The model under review builds one solid part; all positions refer to its coordinate system, in mm. A direction names the side the tool comes from. Coordinates: 2 decimals unless noted, no trailing zeros. Order: outer loops, then holes, each group sorted by start corner. A loop starts at its lowest first (then second) coordinate and runs counter-clockwise, first axis right, second up. Notation, with made-up numbers: M 2,71 L 49,71 A24 cw 49,97 Z; hole C -36.5,18.25 d6. An arc over 180 degrees is marked long. One line per item, written item: value.
Autodesk Inventor part; units mm, degrees
ref_plane "Offsets" through (0, 0, 50) normal (0, 0, 1) x (1, 0, 0)
ref_plane "Work Plane3" through (0, 17, 100) normal (0, 1, 0) x (-1, 0, 0)
ref_plane "YZ Plane" through (0, 0, 0) normal (1, 0, 0) x (0, 1, 0)
ref_plane "Offsets" through (0, 0, 50) normal (0, 0, 1) x (1, 0, 0)
ref_plane "Work Plane4" through (0, 0, 25) normal (0, 0, 1) x (1, 0, 0)
sketch "Sketch1" plane through (0, 0, 0) normal (0, 0, 1) x (1, 0, 0)
  circle A0 centre (0, 0) radius 19.0246
  dimension "d0" = 38.0492
extrude "Extrusion1" add sketch "Sketch1" along normal blind 100
sketch "Sketch2" plane through (0, 0, 100) normal (0, 0, 1) x (1, 0, 0)
  circle A0 centre (0, 0) radius 19.0246
  circle A1 centre (0, 0) radius 17
  dimension "d3" = 34
extrude "Extrusion2" cut sketch "Sketch2" against normal up to surface (75 mm away)
sketch "Sketch8" plane through (0, 0, 100) normal (0, 0, 1) x (1, 0, 0)
  circle A0 centre (0, 0) radius 17
  circle A1 centre (0, 0) radius 12.5
  dimension "d75" = 25
extrude "Extrusion7" cut sketch "Sketch8" against normal up to surface (50 mm away)
sketch "Sketch3" plane through (0, 0, 0) normal (0, 0, -1) x (-1, 0, 0)
  circle A0 centre (0, 0) radius 19.0246
hole "Hole1" at (0, 0, 0) direction (0, 0, 1) diameter 12 depth 50 tip angle 118
sketch "Sketch4" plane through (0, 0, 0) normal (0, 1, 0) x (-1, 0, 0)
  line L0 (-19.0246, 0) -> (19.0246, 0)
  line L1 (3.25, 44.15) -> (3.25, 30.65)
  line L2 (-3.25, 30.65) -> (-3.25, 44.15)
  arc A0 (-3.25, 30.65) -> (3.25, 30.65) centre (0, 30.65) ccw
  arc A1 (3.25, 44.15) -> (-3.25, 44.15) centre (0, 44.15) ccw
  line L3 (0, -9.83) -> (0, 58.98)
  line L4 (-5, 44.15) -> (-5, 30.65)
  arc A2 (-5, 30.65) -> (5, 30.65) centre (0, 30.65) ccw
  line L5 (5, 30.65) -> (5, 44.15)
  arc A3 (5, 44.15) -> (-5, 44.15) centre (0, 44.15) ccw
  point P0 (-19.0246, 25.4)
  point P1 (19.0246, 25.4)
  dimension "d13" = 6.5
  dimension "d15" = 20
  dimension "d76" = 5
extrude "Extrusion3" cut sketch "Sketch4" along normal through all both and the other way through all contours L1 A0 L3 A1 | L3 A0 L2 A1
sketch "Sketch9" plane through (0, 0, 0) normal (0, 0, -1) x (-1, 0, 0)
  circle A0 centre (0, 0) radius 19.0246
  circle A1 centre (0, 0) radius 12.7 construction
  point P0 (-12.7, 0)
  dimension "d49" = 25.4
hole "Hole3" at (12.7, 0, 0) direction (0, 0, 1) diameter 3.937 depth 19.05 tip angle 118
pattern_circular "Circular Pattern1" count 4 over 360 about axis through (0, 0, 25) along (0, 0, -1) of "Hole3"
ref_plane "Work Plane3" through (0, 17, 100) normal (0, 1, 0) x (-1, 0, 0)
extrude "Extrusion12" cut sketch "Sketch4" against normal blind 5 from surface at 17
sketch "Sketch12" plane through (0, 0, 100) normal (0, 0, 1) x (1, 0, 0)
  circle A0 centre (0, 0) radius 10
  circle A1 centre (0, 0) radius 9
  line L0 (-3.0902, 9.5106) -> (-3.0902, 8.4529) construction
  line L1 (3.0902, 9.5106) -> (3.0902, 8.4529) construction
  line L2 (-3.0902, 9.5106) -> (0, 0)
  line L3 (0, 0) -> (3.0902, 9.5106)
  point P0 (2.7812, 8.5595)
  point P1 (-2.7812, 8.5595)
  dimension "d85" = 20
  dimension "d98" = 18
  dimension "d112" = 36
sketch "Sketch15" plane through (0, 0, 100) normal (0, 0, 1) x (1, 0, 0)
  circle A0 centre (0, 0) radius 12
  circle A1 centre (0, 0) radius 12.5
  dimension "d113" = 24
extrude "Extrusion15" cut sketch "Sketch15" against normal blind 12
thread "Thread1"
extrude "Extrusion13" add sketch "Sketch12" along normal blind 14.5 contours L3 L2 A1 | A1 L2 L3
extrude "Extrusion14" add sketch "Sketch12" along normal up to surface (14.5 mm away) contours L3 A1 L2 A0 picked at (1.6921, 9.4688)
pattern_circular "Circular Pattern2" count 5 over 360 about axis through (0, 0, -10) along (0, 0, 1) of "Extrusion14"
sketch "Sketch14" plane through (0, 0, 114.5) normal (0, 0, 1) x (1, 0, 0)
  point P0 (0, 0)
  point P1 (0, 0)
  point P2 (0, 0)
hole "Hole6" at (0, 0, 114.5) direction (0, 0, -1) diameter 6.647 depth 22.2 tip angle 118
properties part number "PWTR-0035" material "Stainless Steel, 303"
(1) Mouldability with a two-part tool opening along Y and no side actions: class faces 1 (the cylindrical face through (-14.62, 0.43, 9.66)), 2 (the cylindrical face through (-9.524, 3.048, 107.148)), 3 (the flat face through (-7, 10, 88)), 4 (the cylindrical face through (-6, -8, 107)) as +Y half, -Y half, draft (parallel to the pull), parting line (faces both ways), or undercut.
Geometry results:
face 1: undercut
face 2: +Y half
face 3: draft
face 4: -Y half
(2) We need section A-A, the plane z = 46. State the section outline as (x, y) points.
Geometry results:
outline: M -4.65,12 L -4.65,16.35 A17 ccw -2.67,-16.79 L -2.67,-5.37 A6 cw -2.67,5.37 L -2.67,12 Z; M 2.67,-16.79 A17 ccw 4.65,16.35 L 4.65,12 L 2.67,12 L 2.67,5.37 A6 cw 2.67,-5.37 Z
(3) Tool access review of faces 5 (the cylindrical face through (9.497, 3.132, 107.148)), 6 (the flat face through (-9, 9, 50)), 7 (the cylindrical face through (14.62, -0.43, 9.66)), 8 (the cylindrical face through (0.11, 14.54, 25.65)), 9 (the cylindrical face through (-0.1, 8.5, 27.4)): name each direction out of +Z, -Z, +X, -X, +Y, -Y from which nothing blocks a thin tool from reaching the whole face with its end or side.
Geometry results:
face 5: +Z, +X, +Y
face 6: +Z
face 7: -Z
face 8: +Y
face 9: +Y, -Y
(4) For L1, parallel to Y at x = 0, z = 7; L2, parallel to X at y = -11.5, z = 37; L3, parallel to Y at x = 0, z = 109, list the stretches that pass through material, from the lowest coordinate up.
Geometry results:
L1: y = -19.02 to -14.67, -10.73 to -6, 6 to 10.73, 14.67 to 19.02
L2: x = -12.52 to -3.25, 3.25 to 12.52
L3: y = -9 to -3.32, 3.32 to 10
(5) We need section B-B, the plane z = 104. State the section outline as (x, y) points, plus the area to 3 significant figures.
Geometry results:
outline: M -10,0 L -9,0 A9 ccw -7.28,-5.29 L -8.09,-5.88 A10 ccw -3.09,-9.51 L -2.78,-8.56 A9 ccw 2.78,-8.56 L 3.09,-9.51 A10 ccw 8.09,-5.88 L 7.28,-5.29 A9 ccw 9,0 L 10,0 A10 ccw 8.09,5.88 L 7.28,5.29 A9 ccw 2.78,8.56 L 3.09,9.51 A10 ccw -3.09,9.51 L -2.78,8.56 A9 ccw -7.28,5.29 L -8.09,5.88 A10 ccw Z; hole C 0,0 d6.65
area: 250 mm2
(6) Insertion check: pin 1 Ø3 at (y, z) = (8, 30) entering from -X; pin 2 Ø5 at (x, y) = (0, -12.7) entering from -Z; pin 3 Ø6 at (x, y) = (0, 0) entering from +Z; pin 4 Ø3 at (y, z) = (-1.5, 31.5) entering from -X. Each pin has a flat end and moves straight along its axis. Give the tip position at first contact, or say it passes through.
Geometry results:
pin 1: stops at x = -15.71
pin 2: stops at z = 0
pin 3: stops at z = 92.11
pin 4: stops at x = -17
